For this review, take the finished solid that the model builds, in its own axes (mm). Face numbers are marked on the shaded views. A direction names the side the tool comes from. Round coordinates to 2 decimals unless told otherwise and drop trailing zeros. Write each loop counter-clockwise with the first axis right and the second up, starting at its lowest first coordinate (ties: lowest second). Pieces come first, ordered by that corner, then holes. Notation, with made-up numbers: (-23, 0) -> (15, 0) arc R24 cw to (15, 24) -> close; hole circle Ø6 at (-36.75, 16). An arc over 180 degrees is marked (long way). Answer in a Markdown table with one row per item. Add a question column.
```python
from build123d import *

# Parameters (mm, degrees)
CUT_EXTRUDE1_DEPTH      = 9.717797887
CUT_EXTRUDE1_DEPTH_BACK = 9.717797887
SKETCH2_R               = 1.5
FILLET2_R               = 0.2


with BuildPart() as part:
    # Sketch1 → Revolve1 (revolve)
    with BuildSketch(Plane.XY, mode=Mode.PRIVATE) as revolve1_sk:
        Polygon((0, 5), (-2, 6), (-2, 0), (2, 0), (2, 6), align=None)
    revolve(revolve1_sk.sketch.rotate(Axis((-9.793827425, 0, 0), (1, 0, 0)), 90), axis=Axis((-9.793827425, 0, 0), (1, 0, 0)))

    # Sketch2 → Cut-Extrude1 (cut, two sides: drawn at the far end of the back side and taken through both)
    with BuildSketch(Plane(origin=(0, 0, 0), x_dir=(0, 0, -1), z_dir=(1, 0, 0)).offset(-CUT_EXTRUDE1_DEPTH_BACK)):
        Circle(SKETCH2_R)
    extrude(amount=CUT_EXTRUDE1_DEPTH + CUT_EXTRUDE1_DEPTH_BACK, mode=Mode.SUBTRACT)

    # Fillet2
    fillet2_edges = [part.edges().sort_by_distance(p)[0] for p in [
        (-2, 0, -6),
        (2, 0, -6),
    ]]
    fillet(fillet2_edges, radius=FILLET2_R)


solid = part.part
```
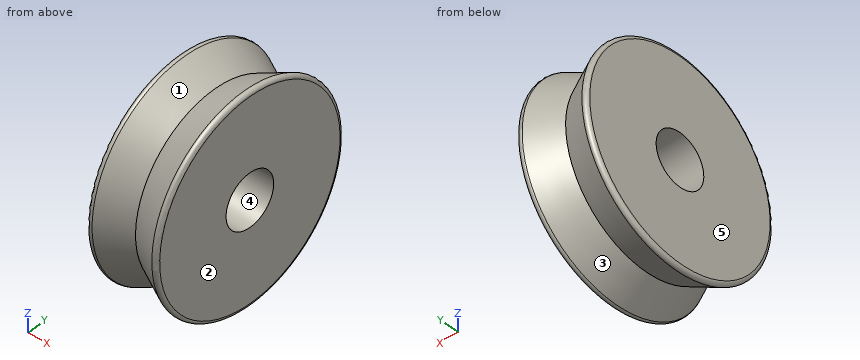
1. Clearance check with flat-ended pins moving along their axes: pin 1 Ø2.5 at (y, z) = (0, 0) entering from +X; pin 2 Ø2 at (x, y) = (-1, 1.5) entering from -Z. State where each tip first meets the part, or that it passes through.
2. The part is to be moulded in two halves that separate along X. For the marked faces 3, 4 and 5, say which applies: pulls with the +X half, pulls with the -X half, needs draft (parallel to the pull), parting line crosses it, or undercut.
3. We need section A-A (z = 0). Write out the cut boundary in (x, y).
4. For L1, parallel to Y at x = -1.75, z = -0.5; L2, parallel to X at y = 4, z = 3.5; L3, parallel to X at y = 4.5, z = 3, list the stretches that pass through material, from the lowest coordinate up. Write a range as [from, to].
5. We need section C-C (x = 1). Write out the cut boundary in (y, z), plus the area to 3 significant figures.
6. Tool access review of the marked faces 1 and 2: name each direction out of +Z, -Z, +X, -X, +Y, -Y from which nothing blocks a thin tool from reaching the whole face with its end or side.
Response:
| question | item | result |
|---|---|---|
| 1 | pin 1 | through |
| 1 | pin 2 | z = -5.81 |
| 2 | face 3 | undercut |
| 2 | face 4 | needs draft |
| 2 | face 5 | pulls with the -X half |
| 3 | outline | (-2, -5.68) arc R0.2 ccw to (-1.71, -5.86) -> (0, -5) -> (1.71, -5.86) arc R0.2 ccw to (2, -5.68) -> (2, -1.5) -> (-2, -1.5) -> close; (-2, 1.5) -> (2, 1.5) -> (2, 5.68) arc R0.2 ccw to (1.71, 5.86) -> (0, 5) -> (-1.71, 5.86) arc R0.2 ccw to (-2, 5.68) -> close |
| 4 | L1 | [-5.85, -1.41], [1.41, 5.85] |
| 4 | L2 | [-2, -0.63], [0.63, 2] |
| 4 | L3 | [-2, -0.82], [0.82, 2] |
| 5 | outline | circle Ø11 at (0, 0); hole circle Ø3 at (0, 0) |
| 5 | area | 88.0 mm2 |
| 6 | face 1 | none |
| 6 | face 2 | +Z, -Z, +X, +Y, -Y |
